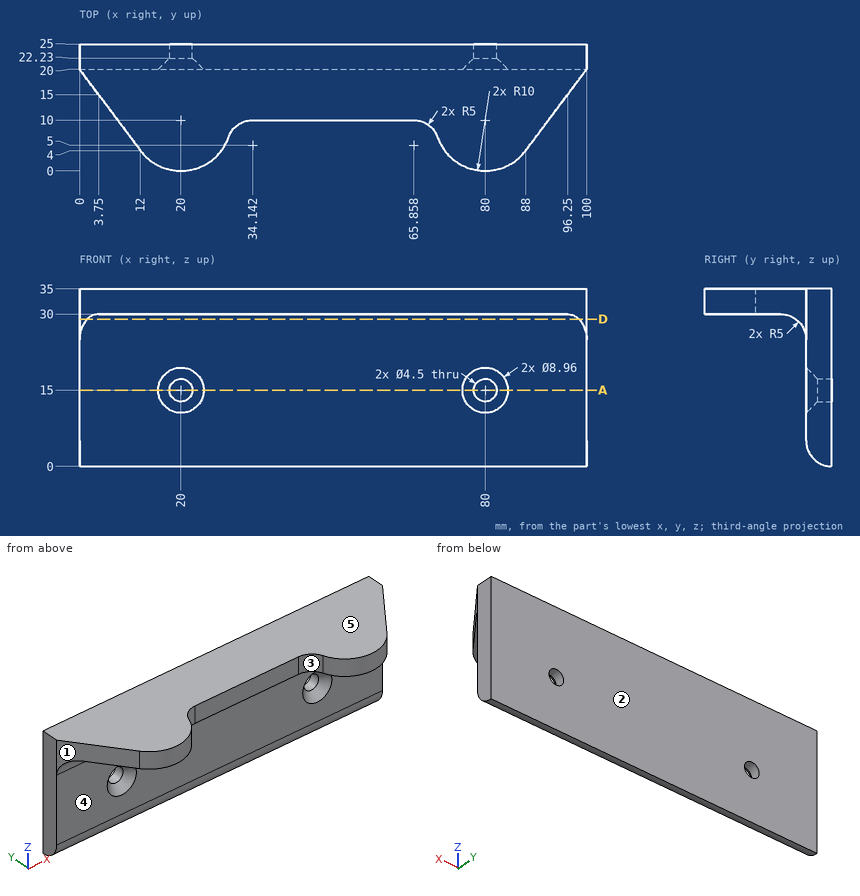
Design review of the part shown in the three views and the two pictorial views. Dimensions are in mm from the part's minimum x, y and z. A direction names the side the tool comes from. Round coordinates to 2 decimals unless told otherwise and drop trailing zeros. Loops run counter-clockwise (first coordinate to the right, second up) from the corner with the lowest first, then second, coordinate; pieces in that order, holes last.
1) The part is to be moulded in two halves that separate along X. For the marked faces 1, 2 and 3, say which applies: pulls with the +X half, pulls with the -X half, needs draft (parallel to the pull), parting line crosses it, or undercut.
Values follow:
face 1: pulls with the -X half
face 2: needs draft
face 3: undercut
2) Consider section A-A on z = 15. State the section outline as (x, y) points, then the cut area to 3 significant figures.
Values follow:
outline: (0, 20) - (15.52, 20) - (17.75, 22.23) - (17.75, 25) - (0, 25) - close; (22.25, 22.23) - (24.48, 20) - (75.52, 20) - (77.75, 22.23) - (77.75, 25) - (22.25, 25) - close; (82.25, 22.23) - (84.48, 20) - (100, 20) - (100, 25) - (82.25, 25) - close
area: 445 mm2
3) Consider section D-D on z = 29. State the section outline as (x, y) points.
Values follow:
outline: (0, 20) - (1.5, 18) - (98.5, 18) - (100, 20) - (100, 25) - (0, 25) - close
4) Clearance check with flat-ended pins moving along their axes: P1, Ø1, axis at y = 18, z = 25.5, coming from the -X side; P2, Ø6, axis at x = 80, z = 15, coming from the -Y side; P3, Ø5.5, axis at x = 56, z = 33.5, coming from the -Y side; P4, Ø4.5, axis at x = 44, y = 10.5, coming from the -Z side. State where each tip first meets the part, or that it passes through.
Values follow:
P1: passes through
P2: stops at y = 21.48
P3: stops at y = 10
P4: stops at z = 30
5) Wall thickness on line 1 along X through (y, z) = (24.25, 15); line 2 along Z through (x, y) = (62, 10.75); line 3 along Y through (x, z) = (57, 5): over which ranges is each line inside the solid? List them lowest first.
Values follow:
line 1: x = 0 to 17.75, 22.25 to 77.75, 82.25 to 100
line 2: z = 30 to 35
line 3: y = 20 to 25
6) Tool access review of the marked faces 4 and 5: name each direction out of +Z, -Z, +X, -X, +Y, -Y from which nothing blocks a thin tool from reaching the whole face with its end or side.
Values follow:
face 4: -Z, +X, -X, -Y
face 5: +Z, +X, -X, +Y, -Y
